Check sheet for the modelled part. Datum: model origin and axes. Units: mm. A direction names the side the tool comes from. Coordinates: 2 decimals unless noted, no trailing zeros. Write each loop counter-clockwise with the first axis right and the second up, starting at its lowest first coordinate (ties: lowest second). Pieces come first, ordered by that corner, then holes. Notation, with made-up numbers: (-0.75, -37) - (25.25, -37) arc R10 ccw to (25.25, -22) - close; hole circle Ø4 at (70, -17). An arc over 180 degrees is marked (long way). Use one line per item in the form item = value. Start each with the question number.
1. Go/stop test with flat-tipped pins: pin 1 Ø12 at (y, z) = (-11, 21.5) entering from -X (3 decimals); pin 2 Ø2 at (x, y) = (-12, -15.5) entering from +Z; pin 3 Ø24 at (x, z) = (0, 0) entering from +Y. Record where each tip stops, or that it passes through.
2. Cross-section at C-C on z = 0. Record the boundary of the cut face in (x, y), then the cut area to 3 significant figures.
3. Cross-section at A-A on x = 0. Record the boundary of the cut face in (y, z).
4. Cross-section at B-B on y = -43. Record the boundary of the cut face in (x, z).
5. Scan lines: line 1 along Z through (x, y) = (0, -45.5); line 2 along Z through (x, y) = (0, -18); line 3 along Y through (x, z) = (-5.5, 12). Record each from-to range of solid material in increasing order.
6. Cross-section at D-D on y = -26.5. Record the boundary of the cut face in (x, z), then the cut area to 3 significant figures.
7. Tool access check on faces 1 (the face through (0, -25, 30)), 2 (the face through (-14.985, -46.056, 0.66)). Record the directions out of +Z, -Z, +X, -X, +Y, -Y that give a thin tool (end or side, any length) a straight path to the whole face; none if there is none.
8. Draft check along X on faces 3 (the face through (-14.985, -3.944, 0.66)), 4 (the face through (-9, 0, -13)), 5 (the face through (-12.42, -49.7, 19.63)), 6 (the face through (-4, -8, 7)). Enter one of: +X half, -X half, draft (parallel to the pull), parting line (faces both ways), or undercut.
```python
from build123d import *

# Parameters (mm, degrees)
F0_W     = 40
F0_H     = 60
F0_R     = 15
F0_R_2   = 7.5
F1_DEPTH = 50
F2_DEPTH = 8
F3_R     = 15
F4_DEPTH = 8
F5_SIZE2 = 20
F5_SIZE  = 15
F6_R     = 1


with BuildPart() as f1:
    # F0 (on Front) → F1 (new body)
    with BuildSketch(Plane.XZ):
        Rectangle(F0_W, F0_H)
        Circle(F0_R, mode=Mode.SUBTRACT)
        Circle(F0_R)
        Circle(F0_R_2, mode=Mode.SUBTRACT)
    extrude(amount=F1_DEPTH)

    # F0 (on Front) → F2 (cut)
    with BuildSketch(Plane.XZ):
        Circle(F0_R)
        Circle(F0_R_2, mode=Mode.SUBTRACT)
    extrude(amount=F2_DEPTH, mode=Mode.SUBTRACT)

    # F3 (on face) → F4 (cut)
    with BuildSketch(Plane.XZ.offset(50)):
        Circle(F3_R)
    extrude(amount=-F4_DEPTH, mode=Mode.SUBTRACT)

    # F5
    f5_edges = [f1.edges().sort_by_distance(p)[0] for p in [
        (20, -25, 30),
        (-20, -25, 30),
    ]]
    f5_side = f1.faces().sort_by_distance((0, -25, 30))[0]
    chamfer(f5_edges, length=F5_SIZE, length2=F5_SIZE2, reference=f5_side)

    # F6
    f6_edges = [f1.edges().sort_by_distance(p)[0] for p in [
        (-5, -25, 30),
        (5, -25, 30),
        (20, -25, 10),
        (-12.5, 0, 20),
        (0, 0, 30),
        (12.5, 0, 20),
        (12.5, -50, 20),
        (-12.5, -50, 20),
        (0, -50, 30),
        (-20, -50, -10),
        (20, -50, -10),
        (20, 0, -10),
        (-20, 0, -10),
        (-20, -25, 10),
    ]]
    fillet(f6_edges, radius=F6_R)


solid = f1.part
```
Final values:
q1.pin_1 = -15.875
q1.pin_2 = 22
q1.pin_3 = -8
q2.outline = (-20, -49) arc R1 ccw to (-19, -50) - (-15, -50) - (-15, -42) - (-7.5, -42) - (-7.5, -8) - (-15, -8) - (-15, 0) - (-19, 0) arc R1 ccw to (-20, -1) - close; (7.5, -42) - (15, -42) - (15, -50) - (19, -50) arc R1 ccw to (20, -49) - (20, -1) arc R1 ccw to (19, 0) - (15, 0) - (15, -8) - (7.5, -8) - close
q2.area = 1,010 mm²
q3.outline = (-50, -30) - (0, -30) - (0, -15) - (-8, -15) - (-8, -7.5) - (-42, -7.5) - (-42, -15) - (-50, -15) - close; (-50, 15) - (-42, 15) - (-42, 7.5) - (-8, 7.5) - (-8, 15) - (0, 15) - (0, 29) arc R1 ccw to (-1, 30) - (-49, 30) arc R1 ccw to (-50, 29) - close
q4.outline = (-20, -30) - (20, -30) - (20, 9.67) arc R1 ccw to (19.8, 10.27) - (5.3, 29.6) arc R1 ccw to (4.5, 30) - (-4.5, 30) arc R1 ccw to (-5.3, 29.6) - (-19.8, 10.27) arc R1 ccw to (-20, 9.67) - close; hole circle Ø30 at (0, 0)
q5.line_1 = -30 to -15, 15 to 30
q5.line_2 = -30 to -7.5, 7.5 to 30
q5.line_3 = -42 to -8
q6.outline = (-20, -30) - (20, -30) - (20, 9.67) arc R1 ccw to (19.8, 10.27) - (5.3, 29.6) arc R1 ccw to (4.5, 30) - (-4.5, 30) arc R1 ccw to (-5.3, 29.6) - (-19.8, 10.27) arc R1 ccw to (-20, 9.67) - close; hole circle Ø15 at (0, 0)
q6.area = 1,920 mm²
q7.face_1 = +Z, +X, -X, +Y, -Y
q7.face_2 = -Y
q8.face_3 = undercut
q8.face_4 = draft
q8.face_5 = -X half
q8.face_6 = undercut
